```python
from build123d import *

# Parameters (mm, degrees)
BOSS_EXTRUDE5_DEPTH = 0.6
BOSS_EXTRUDE6_DEPTH = 1.225
SKETCH15_R          = 0.3
SKETCH17_W          = 5
SKETCH17_H          = 5
CUT_EXTRUDE1_DEPTH  = 10
SKETCH18_W          = 13.5
SKETCH18_H          = 1.2
BOSS_EXTRUDE7_DEPTH = 3


with BuildPart() as part:
    # Sketch1 → Boss-Extrude5 (new body)
    with BuildSketch(Plane(origin=(0, 0, 0), x_dir=(1, 0, 0), z_dir=(0, 1, 0))):
        with BuildLine():
            Line((0.8, 26.4), (19.9, 26.4))
            ThreePointArc((19.9, 26.4), (21.455634919, 25.755634919), (22.1, 24.2))
            Line((22.1, 24.2), (22.1, 0.8))
            ThreePointArc((22.1, 0.8), (21.455634919, -0.755634919), (19.9, -1.4))
            Line((19.9, -1.4), (0.8, -1.4))
            ThreePointArc((0.8, -1.4), (-0.755634919, -0.755634919), (-1.4, 0.8))
            Line((-1.4, 0.8), (-1.4, 24.2))
            ThreePointArc((-1.4, 24.2), (-0.755634919, 25.755634919), (0.8, 26.4))
        make_face()
    extrude(amount=BOSS_EXTRUDE5_DEPTH)

    # Sketch13 → Boss-Extrude6 (add)
    with BuildSketch(Plane(origin=(0, 0.6, 0), x_dir=(1, 0, 0), z_dir=(0, 1, 0))):
        with BuildLine():
            Line((-0.1, 24.2), (-0.1, 0.8))
            ThreePointArc((-0.1, 0.8), (0.163603897, 0.163603897), (0.8, -0.1))
            Line((0.8, -0.1), (19.9, -0.1))
            ThreePointArc((19.9, -0.1), (20.536396103, 0.163603897), (20.8, 0.8))
            Line((20.8, 0.8), (20.8, 24.2))
            ThreePointArc((20.8, 24.2), (20.536396103, 24.836396103), (19.9, 25.1))
            Line((19.9, 25.1), (0.8, 25.1))
            ThreePointArc((0.8, 25.1), (0.163603897, 24.836396103), (-0.1, 24.2))
        make_face()
        with BuildLine():
            Line((19.9, 24.5), (0.8, 24.5))
            ThreePointArc((0.8, 24.5), (0.587867966, 24.412132034), (0.5, 24.2))
            Line((0.5, 24.2), (0.5, 0.8))
            ThreePointArc((0.5, 0.8), (0.587867966, 0.587867966), (0.8, 0.5))
            Line((0.8, 0.5), (19.9, 0.5))
            ThreePointArc((19.9, 0.5), (20.112132034, 0.587867966), (20.2, 0.8))
            Line((20.2, 0.8), (20.2, 24.2))
            ThreePointArc((20.2, 24.2), (20.112132034, 24.412132034), (19.9, 24.5))
        make_face(mode=Mode.SUBTRACT)
    extrude(amount=BOSS_EXTRUDE6_DEPTH)

    # Sweep1: sweep along a path in Sketch16
    with BuildLine(Plane(origin=(0, 1.825, 0), x_dir=(1, 0, 0), z_dir=(0, 1, 0))) as sweep1_path:
        Line((-0.1, 24.2), (-0.1, 0.8))
        ThreePointArc((-0.1, 0.8), (0.163603897, 0.163603897), (0.8, -0.1))
        Line((0.8, -0.1), (19.9, -0.1))
        ThreePointArc((19.9, -0.1), (20.536396103, 0.163603897), (20.8, 0.8))
        Line((20.8, 0.8), (20.8, 24.2))
        ThreePointArc((20.8, 24.2), (20.536396103, 24.836396103), (19.9, 25.1))
        Line((19.9, 25.1), (0.8, 25.1))
        ThreePointArc((0.8, 25.1), (0.163603897, 24.836396103), (-0.1, 24.2))
    # Sketch15 → Sweep1 (sweep)
    with BuildSketch(Plane(origin=(0, 0, -10.5), x_dir=(-1, 0, 0), z_dir=(0, 0, -1))):
        with Locations((-20.8, 1.5)):
            Circle(SKETCH15_R)
    sweep(path=sweep1_path.line)

    # Sketch17 → Cut-Extrude1 (cut)
    with BuildSketch(Plane(origin=(0, 0.6, 0), x_dir=(1, 0, 0), z_dir=(0, 1, 0))):
        with Locations((1.1, 23.9)):
            Rectangle(SKETCH17_W, SKETCH17_H)
        with Locations((19.6, 23.9)):
            Rectangle(SKETCH17_W, SKETCH17_H)
        with Locations((19.6, 1.1)):
            Rectangle(SKETCH17_W, SKETCH17_H)
        with Locations((1.1, 1.1)):
            Rectangle(SKETCH17_W, SKETCH17_H)
    extrude(amount=CUT_EXTRUDE1_DEPTH, mode=Mode.SUBTRACT)

    # Sketch18 → Boss-Extrude7 (add)
    with BuildSketch(Plane(origin=(0, 0.6, 0), x_dir=(1, 0, 0), z_dir=(0, 1, 0))):
        with Locations((10.35, 23.4)):
            Rectangle(SKETCH18_W, SKETCH18_H)
    extrude(amount=BOSS_EXTRUDE7_DEPTH)


solid = part.part
```
Geometry check sheet. Reference: the model listing, model coordinates, mm. A direction names the side the tool comes from. Round coordinates to 2 decimals unless told otherwise and drop trailing zeros. Order: outer loops, then holes, each group sorted by start corner. A loop starts at its lowest first (then second) coordinate and runs counter-clockwise, first axis right, second up. Notation, with made-up numbers: M 53.25,38 L 101.25,38 A14 ccw 101.25,54 Z; hole C -14,70 d10. An arc over 180 degrees is marked long. Answer as CSV lines item,"result".
1) Sectioned sample at D-D on x = 18.5. Record the cut outline in (y, z), and give its area (3 significant figures).
Entries:
outline,"M 0,-26.4 L 0.6,-26.4 L 0.6,1.4 L 0,1.4 Z"
area,"16.7 mm2"
2) Sectioned sample at B-B on z = -5. Record the cut outline in (x, y) (3 decimals).
Entries:
outline,"M -1.4,0 L 22.1,0 L 22.1,0.6 L 20.8,0.6 L 20.8,1.2 A0.3 ccw 20.8,1.8 L 20.8,1.825 L 20.2,1.825 L 20.2,0.6 L 0.5,0.6 L 0.5,1.825 L -0.1,1.825 L -0.1,1.8 A0.3 ccw -0.1,1.2 L -0.1,0.6 L -1.4,0.6 Z"
3) Tool access check on faces 1 (the face through (10, 2, -24)), 2 (the face through (17.1, 2, -23)), 3 (the face through (0.1, 1.2, -3.6)), 4 (the face through (3.6, 1.2, -24.8)), 5 (the face through (0.5, 1, -13)). Record the directions out of +Z, -Z, +X, -X, +Y, -Y that give a thin tool (end or side, any length) a straight path to the whole face; none if there is none.
Entries:
face 1,"+X, -X, +Y"
face 2,"+Z, -Z, +X, +Y"
face 3,"+Z, +X, -X, +Y"
face 4,"+Z, -Z, -X, +Y"
face 5,"+Z, -Z, +Y"
4) Thickness scan on probe 1 along Z at (x, y) = (5.25, 0.7); probe 2 along X at (y, z) = (0.8, -20.5); probe 3 along Y at (x, z) = (9, -1.25). Record the ranges inside material, lowest first. Write a range as [from, to].
Entries:
probe 1,"[-25.1, -24.5], [-24, -22.8], [-0.5, 0.1]"
probe 2,"[-0.1, 0.5], [20.2, 20.8]"
probe 3,"[0, 0.6]"
5) Sectioned sample at A-A on y = 1.5. Record the cut outline in (x, z), and give its area (3 significant figures).
Entries:
outline,"M -0.4,-21.4 L 0.5,-21.4 L 0.5,-3.6 L -0.4,-3.6 Z; M 3.6,-25.4 L 17.1,-25.4 L 17.1,-24.5 L 3.6,-24.5 Z; M 3.6,-24 L 17.1,-24 L 17.1,-22.8 L 3.6,-22.8 Z; M 3.6,-0.5 L 17.1,-0.5 L 17.1,0.4 L 3.6,0.4 Z; M 20.2,-21.4 L 21.1,-21.4 L 21.1,-3.6 L 20.2,-3.6 Z"
area,"72.5 mm2"
6) Sectioned sample at C-C on x = 4.5. Record the cut outline in (y, z) (3 decimals), and give its area (3 significant figures).
Entries:
outline,"M 0,-26.4 L 0.6,-26.4 L 0.6,-25.1 L 1.2,-25.1 A0.3 ccw 1.8,-25.1 L 1.825,-25.1 L 1.825,-24.5 L 0.6,-24.5 L 0.6,-24 L 3.6,-24 L 3.6,-22.8 L 0.6,-22.8 L 0.6,-0.5 L 1.825,-0.5 L 1.825,0.1 L 1.8,0.1 A0.3 ccw 1.2,0.1 L 0.6,0.1 L 0.6,1.4 L 0,1.4 Z"
area,"22.0 mm2"
7) Gauge pin test, flat ends, axial feed: pin 1 Ø0.7 at (y, z) = (1, 0) entering from -X; pin 2 Ø1 at (y, z) = (1.5, -8.5) entering from +X; pin 3 Ø1 at (x, y) = (21, 1.5) entering from -Z. Record the tip position at first contact, or that the pin passes through.
Entries:
pin 1,"x = 3.6"
pin 2,"x = 21.1"
pin 3,"z = -21.4"
8) Mould release check, pull along Z, two halves, no side actions. Record for faces 6 (the face through (20.5, 1.2, -21.4)), 7 (the face through (10, 1, -0.5)), 8 (the face through (-0.74, 0.3, 0.77)): +Z half, -Z half, draft (parallel to the pull), parting line (faces both ways), or undercut.
Entries:
face 6,"-Z half"
face 7,"undercut"
face 8,"+Z half"
